from build123d import *

# Parameters (mm, degrees)
BOSS_EXTRU_1_DEPTH      = 19
CONG_1_R                = 3
ESQUISSE1_R             = 1
BOSS_EXTRU_2_DEPTH      = 2.7
ESQUISSE2_R             = 2
ESQUISSE2_R_2           = 1
ENL_V_MAT_EXTRU_1_DEPTH = 1
CHANFREIN1_SIZE         = 2
CONG_2_R                = 2


with BuildPart() as part:
    # Model → Boss.-Extru.1 (new body)
    with BuildSketch(Plane.XY):
        Polygon((-25.928539703, 10.301582208), (76.096991945, 69.210096437), (141.828136311, 86.310332452), (158.934643692, 22.435471273), (100.081941761, 6.672683012), (-8.057042666, -55.858487698), (-177.373873722, -55.858487698), (-177.373873722, -50.687645053), (-177.373873722, 10.291172324), align=None)
        Polygon((-25.124548608, 7.301637465), (-174.373873722, 7.291378528), (-174.373873722, -50.687645053), (-174.373873722, -52.858487698), (-8.861972593, -52.858487698), (98.923133978, 9.468053786), (155.26069475, 24.557200291), (139.700811798, 82.657041562), (77.245358051, 66.408990356), align=None, mode=Mode.SUBTRACT)
    extrude(amount=BOSS_EXTRU_1_DEPTH)

    # Congé1
    cong_1_edges = [part.edges().sort_by_distance(p)[0] for p in [
        (76.096991945, 69.210096437, 9.5),
        (141.828136311, 86.310332452, 9.5),
        (158.934643692, 22.435471273, 9.5),
        (100.081941761, 6.672683012, 9.5),
        (-8.057042666, -55.858487698, 9.5),
        (-177.373873722, -55.858487698, 9.5),
        (-177.373873722, 10.291172324, 9.5),
        (-25.928539703, 10.301582208, 9.5),
    ]]
    fillet(cong_1_edges, radius=CONG_1_R)

    # Esquisse1 → Boss.-Extru.2 (add)
    with BuildSketch(Plane.XY):
        Polygon((-25.124548608, 7.301637465), (-174.373873722, 7.291378528), (-174.373873722, -50.687645053), (-174.373873722, -52.858487698), (-8.861972593, -52.858487698), (98.923133978, 9.468053786), (155.26069475, 24.557200291), (139.700811798, 82.657041562), (77.245358051, 66.408990356), align=None)
        with Locations(Location((-114.259444544, -13.418125698, 0), (0, 0, 180))):
            Circle(ESQUISSE1_R, mode=Mode.SUBTRACT)
        with Locations(Location((-114.030844544, -32.493525698, 0), (0, 0, 180))):
            Circle(ESQUISSE1_R, mode=Mode.SUBTRACT)
        with Locations(Location((-29.702844544, -2.648525698, 0), (0, 0, 180))):
            Circle(ESQUISSE1_R, mode=Mode.SUBTRACT)
        with Locations(Location((-10.652844544, -46.438125698, 0), (0, 0, 180))):
            Circle(ESQUISSE1_R, mode=Mode.SUBTRACT)
        with Locations(Location((80.685555456, 58.489274302, 0), (0, 0, 180))):
            Circle(ESQUISSE1_R, mode=Mode.SUBTRACT)
        with Locations(Location((92.877555456, 28.085474302, 0), (0, 0, 180))):
            Circle(ESQUISSE1_R, mode=Mode.SUBTRACT)
    extrude(amount=BOSS_EXTRU_2_DEPTH)

    # Esquisse2 → Enlèv. mat.-Extru.1 (cut)
    # profile 1 of 6: a face of its own
    with BuildSketch(Plane(origin=(0, 0, 0), x_dir=(-1, 0, 0), z_dir=(0, 0, -1))):
        with Locations((-80.685555456, 58.489274302)):
            Circle(ESQUISSE2_R)
        with Locations((-80.685555456, 58.489274302)):
            Circle(ESQUISSE2_R_2, mode=Mode.SUBTRACT)
    # profile 2 of 6: a face of its own
    with BuildSketch(Plane(origin=(0, 0, 0), x_dir=(-1, 0, 0), z_dir=(0, 0, -1))):
        with Locations((-92.877555456, 28.085474302)):
            Circle(ESQUISSE2_R)
        with Locations((-92.877555456, 28.085474302)):
            Circle(ESQUISSE2_R_2, mode=Mode.SUBTRACT)
    # profile 3 of 6: a face of its own
    with BuildSketch(Plane(origin=(0, 0, 0), x_dir=(-1, 0, 0), z_dir=(0, 0, -1))):
        with Locations((29.702844544, -2.648525698)):
            Circle(ESQUISSE2_R)
        with Locations((29.702844544, -2.648525698)):
            Circle(ESQUISSE2_R_2, mode=Mode.SUBTRACT)
    # profile 4 of 6: a face of its own
    with BuildSketch(Plane(origin=(0, 0, 0), x_dir=(-1, 0, 0), z_dir=(0, 0, -1))):
        with Locations((10.652844544, -46.438125698)):
            Circle(ESQUISSE2_R)
        with Locations((10.652844544, -46.438125698)):
            Circle(ESQUISSE2_R_2, mode=Mode.SUBTRACT)
    # profile 5 of 6: a face of its own
    with BuildSketch(Plane(origin=(0, 0, 0), x_dir=(-1, 0, 0), z_dir=(0, 0, -1))):
        with Locations((114.259444544, -13.418125698)):
            Circle(ESQUISSE2_R)
        with Locations((114.259444544, -13.418125698)):
            Circle(ESQUISSE2_R_2, mode=Mode.SUBTRACT)
    # profile 6 of 6: a face of its own
    with BuildSketch(Plane(origin=(0, 0, 0), x_dir=(-1, 0, 0), z_dir=(0, 0, -1))):
        with Locations((114.030844544, -32.493525698)):
            Circle(ESQUISSE2_R)
        with Locations((114.030844544, -32.493525698)):
            Circle(ESQUISSE2_R_2, mode=Mode.SUBTRACT)
    extrude(amount=-ENL_V_MAT_EXTRU_1_DEPTH, mode=Mode.SUBTRACT)

    # Chanfrein1
    chanfrein1_edges = [part.edges().sort_by_distance(p)[0] for p in [
        (-100.55320226, 10.296452739, 19),
        (25.256413626, 39.855258654, 19),
        (107.717763914, 77.436374389, 19),
        (-177.373873722, -22.783554585, 19),
        (-91.617923158, -55.858487698, 19),
        (46.189388475, -24.49058773, 19),
        (128.250722147, 14.217256264, 19),
        (150.378629519, 54.383209367, 19),
        (-176.495266971, 9.412625963, 19),
        (-176.495194066, -54.979808041, 19),
        (-8.084540154, -55.756003669, 19),
        (157.858595311, 23.056896097, 19),
        (141.210432656, 85.249539366, 19),
        (76.107372343, 69.184776466, 19),
        (-25.955930978, 10.403787708, 19),
        (100.091914608, 6.648625697, 19),
    ]]
    chamfer(chanfrein1_edges, length=CHANFREIN1_SIZE)

    # Congé2
    cong_2_edges = [part.edges().sort_by_distance(p)[0] for p in [
        (-100.55320226, 10.296452739, 0),
        (25.256413626, 39.855258654, 0),
        (107.717763914, 77.436374389, 0),
        (150.378629519, 54.383209367, 0),
        (128.250722147, 14.217256264, 0),
        (46.189388475, -24.49058773, 0),
        (-91.617923158, -55.858487698, 0),
        (-177.373873722, -22.783554585, 0),
        (-176.495266971, 9.412625963, 0),
        (-176.495194066, -54.979808041, 0),
        (-8.084540154, -55.756003669, 0),
        (157.858595311, 23.056896097, 0),
        (141.210432656, 85.249539366, 0),
        (76.107372343, 69.184776466, 0),
        (-25.955930978, 10.403787708, 0),
        (100.091914608, 6.648625697, 0),
    ]]
    fillet(cong_2_edges, radius=CONG_2_R)


solid = part.part
Build history of the part. All positions in model axes, mm. A direction names the side the tool comes from. Give positions to 0.01 mm unless a question says otherwise; leave off trailing zeros. Write each loop counter-clockwise with the first axis right and the second up, starting at its lowest first coordinate (ties: lowest second). Pieces come first, ordered by that corner, then holes. Notation, with made-up numbers: (-29, 55.5) - (-7, 55.5) arc R18 ccw to (-7, 62.5) - close; hole circle Ø4 at (74.25, 67.25). An arc over 180 degrees is marked (long way). Use one line per item in the form item = value. Start each with the question number.
1. Band-saw the part on A-A on z = 5.75. Write the cut outline in (x, y).
2. Drop flat-ended pins along their axis: pin 1 Ø2 at (y, z) = (22, 10.5) entering from -X; pin 2 Ø4.5 at (x, y) = (-10.65, -46.44) entering from +Z; pin 3 Ø6 at (y, z) = (-23.5, 7.5) entering from +X. Give the stop position or say it passes through.
3. Probe line 1 (Y direction, x = -53, z = 4); line 2 (Z direction, x = 90.5, y = 22); line 3 (X direction, y = 27, z = 11). List the from-to ranges inside material, lowest first. Write a range as [from, to].
4. Two-plate mould, pull along Y, no slides. Class faces 3 (the face through (128.385, 15.274, 17.986)), 4 (the face through (26.25, 39.77, 0.6)), 5 (the face through (-174.374, -23, 11)), 6 (the face through (-12, 1, 2.7)): released by +Y, released by -Y, zero draft, split by the parting line, or undercut.
5. 3-axis set-ups, long thin cutter, end or side, ignore diameter. For faces 1 (the face through (26.78, 37.27, 10.74)), 2 (the face through (107.281, 77.323, 9.395)): which of +Z, -Z, +X, -X, +Y, -Y reach the whole face in a straight line?
Conclusion:
q1.outline = (-177.37, -52.86) arc R3 ccw to (-174.37, -55.86) - (-8.86, -55.86) arc R3 ccw to (-7.36, -55.46) - (99.74, 6.47) arc R3 cw to (100.46, 6.78) - (156.04, 21.66) arc R3 ccw to (158.16, 25.33) - (142.6, 83.43) arc R3 ccw to (138.95, 85.56) - (76.49, 69.31) arc R3 ccw to (75.75, 69.01) - (-25.23, 10.7) arc R3 cw to (-26.73, 10.3) - (-174.37, 10.29) arc R3 ccw to (-177.37, 7.29) - close; hole (-174.37, -52.86) - (-8.86, -52.86) - (98.92, 9.47) - (155.26, 24.56) - (139.7, 82.66) - (77.25, 66.41) - (-25.12, 7.3) - (-174.37, 7.29) - close
q2.pin_1 = -7.4
q2.pin_2 = 2.7
q2.pin_3 = 53.09
q3.line_1 = [-55.86, -52.86], [7.3, 10.3]
q3.line_2 = [0, 2.7]
q3.line_3 = [2.99, 8.99], [154.61, 157.71]
q4.face_3 = released by -Y
q4.face_4 = released by +Y
q4.face_5 = undercut
q4.face_6 = undercut
q5.face_1 = +Z
q5.face_2 = +Z, -Z, -X, +Y
